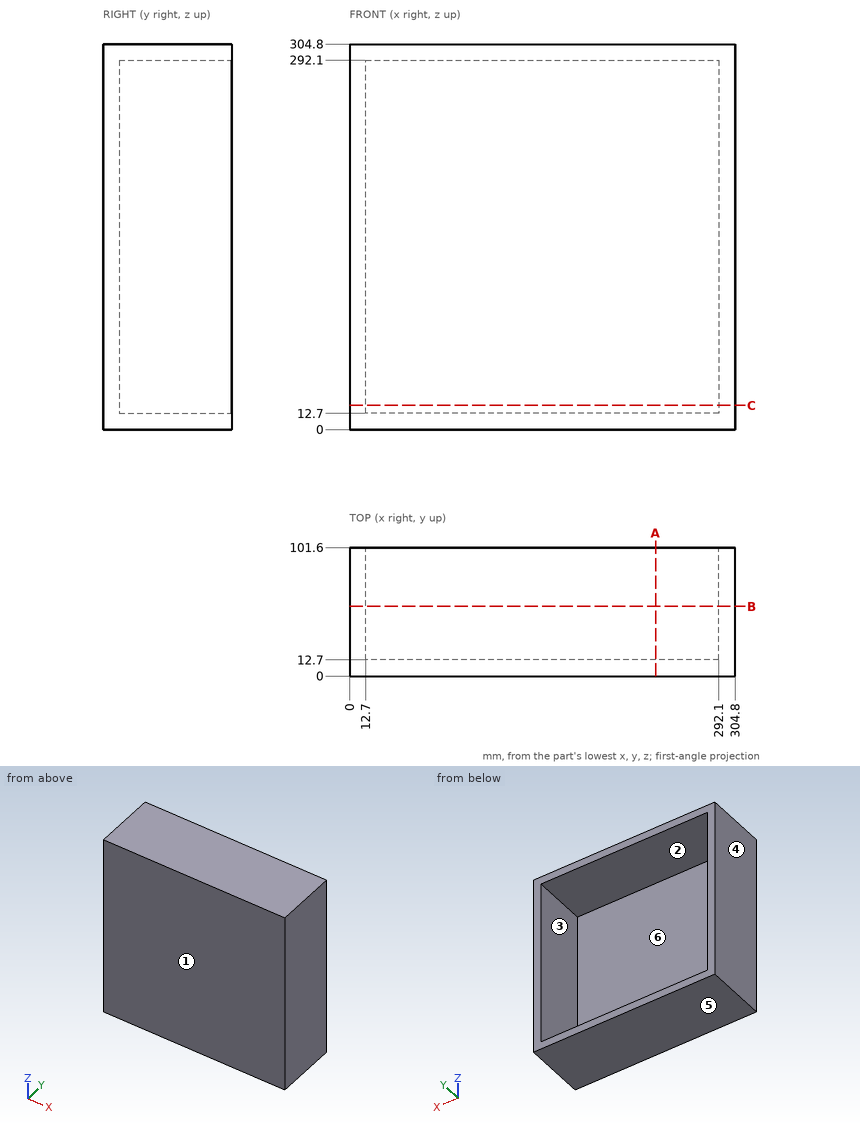
Check sheet for the drawn part. Datum: minimum x, y, z corner. Units: mm. A direction names the side the tool comes from. Round coordinates to 2 decimals unless told otherwise and drop trailing zeros. Order: outer loops, then holes, each group sorted by start corner. A loop starts at its lowest first (then second) coordinate and runs counter-clockwise, first axis right, second up. Notation, with made-up numbers: (36, -20.5) - (89, -20.5) arc R23 cw to (89, 1.5) - close; hole circle Ø3 at (10, 29.5). An arc over 180 degrees is marked (long way). Use a Markdown table: item, result. Add a question column.
(1) Material ranges on line 1 along Z through (x, y) = (233.5, 19.5); line 2 along Y through (x, z) = (41.5, 16.5), recorded low to high. Write a range as [from, to].
(2) Sectioned sample at A-A, the plane x = 242. Enter the section's corners in (y, z).
(3) Release check for a two-part mould opening along X. For the marked faces 1, 2, 3 and 4 record: pulls with the +X half, pulls with the -X half, needs draft (parallel to the pull), parting line crosses it, or undercut.
(4) Sectioned sample at B-B, the plane y = 55. Enter the section's corners in (x, z), and give its area (3 significant figures).
(5) Sectioned sample at C-C, the plane z = 19. Enter the section's corners in (x, y), and give its area (3 significant figures).
(6) Depth check by flat-ended pin: pin 1 (3 mm diameter, centred on x = 98, z = 78, fed in from +Y). Enter the tip coordinate at first touch or a pass-through.
(7) Tool access check on the marked faces 5 and 6. Record the directions out of +Z, -Z, +X, -X, +Y, -Y that give a thin tool (end or side, any length) a straight path to the whole face; none if there is none.
Answers below:
| question | item | result |
|---|---|---|
| 1 | line 1 | [0, 12.7], [292.1, 304.8] |
| 1 | line 2 | [0, 12.7] |
| 2 | outline | (0, 0) - (101.6, 0) - (101.6, 12.7) - (12.7, 12.7) - (12.7, 292.1) - (101.6, 292.1) - (101.6, 304.8) - (0, 304.8) - close |
| 3 | face 1 | needs draft |
| 3 | face 2 | undercut |
| 3 | face 3 | undercut |
| 3 | face 4 | pulls with the -X half |
| 4 | outline | (0, 0) - (304.8, 0) - (304.8, 304.8) - (0, 304.8) - close; hole (12.7, 12.7) - (292.1, 12.7) - (292.1, 292.1) - (12.7, 292.1) - close |
| 4 | area | 14,800 mm² |
| 5 | outline | (0, 0) - (304.8, 0) - (304.8, 101.6) - (292.1, 101.6) - (292.1, 12.7) - (12.7, 12.7) - (12.7, 101.6) - (0, 101.6) - close |
| 5 | area | 6,130 mm² |
| 6 | pin 1 | y = 12.7 |
| 7 | face 5 | -Z, +X, -X, +Y, -Y |
| 7 | face 6 | +Y |
